Autodesk Inventor part; units mm, degrees
ref_plane "YZ Plane" through (0, 0, 0) normal (1, 0, 0) x (0, 1, 0)
ref_plane "XZ Plane" through (0, 0, 0) normal (0, 1, 0) x (-1, 0, 0)
ref_plane "XY Plane" through (0, 0, 0) normal (0, 0, 1) x (1, 0, 0)
sketch "Sketch1" plane through (0, 0, 0) normal (0, 1, 0) x (-1, 0, 0)
  line L0 (-24.05, -31.5) -> (24.05, -31.5)
  line L1 (24.05, -31.5) -> (24.05, 31.5)
  line L2 (24.05, 31.5) -> (-24.05, 31.5)
  line L3 (-24.05, 31.5) -> (-24.05, -31.5)
  line L4 (-24.05, -31.5) -> (24.05, 31.5) construction
  line L5 (24.05, -31.5) -> (-24.05, 31.5) construction
  point P0 (0, 0)
  dimension "d0" = 63
  dimension "d1" = 48.1
extrude "Extrusion1" add sketch "Sketch1" along normal blind 1
sketch "Sketch2" plane through (0, 1, 0) normal (0, 1, 0) x (1, 0, 0)
  line L0 (-24.05, -31.5) -> (24.05, -31.5)
  line L1 (-24.05, -31.5) -> (24.05, -31.5)
  line L2 (24.05, -31.5) -> (24.05, -33)
  line L3 (24.05, -33) -> (-24.05, -33)
  line L4 (-24.05, -33) -> (-24.05, -31.5)
  line L5 (-24.05, 31.5) -> (24.05, 31.5)
  line L6 (24.05, 31.5) -> (24.05, 33)
  line L7 (24.05, 33) -> (-24.05, 33)
  line L8 (-24.05, 33) -> (-24.05, 31.5)
  point P0 (0, 0)
  point P1 (20.95, -31.5)
  dimension "d4" = 1.5
extrude "Extrusion2" add sketch "Sketch2" against normal blind 25
properties part number "Module Cover"
Model file for the job. Use its own axes, mm. A direction names the side the tool comes from. Give positions to 0.01 mm unless a question says otherwise; leave off trailing zeros. Order: outer loops, then holes, each group sorted by start corner. A loop starts at its lowest first (then second) coordinate and runs counter-clockwise, first axis right, second up. Notation, with made-up numbers: M 85,-29.5 L 100,-29.5 A16 ccw 100,-11.5 Z; hole C 35.5,83 d7. An arc over 180 degrees is marked long. Put each result on its own line as item: value. Start each with the question number.
(1) Band-saw the part on A-A on y = -19.75. Give the cut face in (x, z), then the cut area to 3 significant figures.
(2) Pull direction Z, two halves, no side cores. Call faces 1 (the face through (0, -11, 33)), 2 (the face through (0, -12, -31.5)), 3 (the face through (0, 1, 0)): released by +Z, released by -Z, zero draft, split by the parting line, or undercut.
(3) Drill centre lines: L1, parallel to Z at x = -2, y = -19.25; L2, parallel to Y at x = -18, z = -5. Where is each one in solid material? Low to high. Write a range as [from, to].
(4) Pin check, flat tips, straight feed: pin 1 Ø2 at (y, z) = (-2.5, 6.5) entering from -X; pin 2 Ø14.5 at (x, z) = (9, -3.5) entering from -Y. Stop position of each tip, or through.
(5) Tool access for faces 4 (the face through (0, -11, -33)), 5 (the face through (0, 0, 0)): list every direction of +Z, -Z, +X, -X, +Y, -Y with a clear straight run to the whole face (end or side of a thin tool).
(6) Band-saw the part on B-B on x = -8. Give the cut face in (y, z).
(7) Band-saw the part on C-C on z = 12. Give the cut face in (x, y).
Results below:
1. outline: M -24.05,-33 L 24.05,-33 L 24.05,-31.5 L -24.05,-31.5 Z; M -24.05,31.5 L 24.05,31.5 L 24.05,33 L -24.05,33 Z
1. area: 144 mm2
2. face 1: released by +Z
2. face 2: undercut
2. face 3: zero draft
3. L1: z = [-33, -31.5], [31.5, 33]
3. L2: y = [0, 1]
4. pin 1: passes through
4. pin 2: stops at y = 0
5. face 4: -Z, +X, -X, +Y, -Y
5. face 5: +X, -X, -Y
6. outline: M -24,-33 L 1,-33 L 1,33 L -24,33 L -24,31.5 L 0,31.5 L 0,-31.5 L -24,-31.5 Z
7. outline: M -24.05,0 L 24.05,0 L 24.05,1 L -24.05,1 Z
